Geometry: final body of the model. Coordinates: model frame, mm. Coordinates: 2 decimals unless noted, no trailing zeros. Order: outer loops, then holes, each group sorted by start corner. A loop starts at its lowest first (then second) coordinate and runs counter-clockwise, first axis right, second up. Notation, with made-up numbers: (-5.5, 28) -> (43.5, 28) arc R16 cw to (43.5, 51) -> close; hole circle Ø6 at (-20, -9.5). An arc over 180 degrees is marked (long way). Use one line per item in the form item = value.
```python
from build123d import *

# Parameters (mm, degrees)
EXTRUDE_1_DEPTH = 6


with BuildPart() as part:
    # 스케치1 → 보스-돌출1 (new, symmetric)
    with BuildSketch(Plane(origin=(0, 0, 0), x_dir=(0, 0, -1), z_dir=(1, 0, 0))):
        with BuildLine():
            Line((0, 6), (0, -6))
            Line((0, -6), (-60, -12))
            Line((-60, -12), (-70, -12))
            Line((-70, -12), (-70, -7))
            Line((-70, -7), (-82, -7))
            Line((-82, -7), (-89.403074012, -12))
            Line((-89.403074012, -12), (-149, -12))
            Line((-149, -12), (-149, -20))
            Line((-149, -20), (-199.739657381, -20))
            Line((-199.739657381, -20), (-235.816329231, 20))
            Line((-235.816329231, 20), (-160, 20))
            Line((-160, 20), (-160, 16.749981814))
            Line((-160, 16.749981814), (-156.437513639, 12))
            Line((-156.437513639, 12), (-156.019273901, 12))
            Line((-156.019273901, 12), (-153.375521927, 9.919487169))
            ThreePointArc((-153.375521927, 9.919487169), (-148.913971149, 8.215866364), (-146.000538153, 12))
            Line((-146.000538153, 12), (-60, 12))
            Line((-60, 12), (0, 6))
        make_face()
    extrude(amount=EXTRUDE_1_DEPTH, both=True)


solid = part.part
```
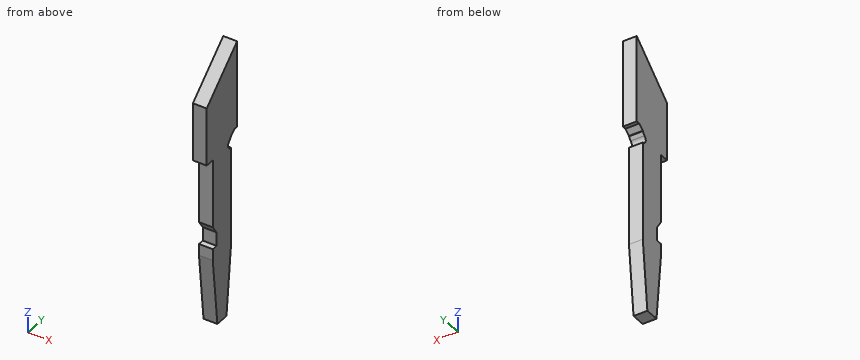
1) Section C-C, the plane y = 4. Output: boundary loops of the cut face in (x, z).
Results found:
outline = (-6, 0) -> (6, 0) -> (6, 221.39) -> (-6, 221.39) -> close
2) Section A-A, the plane x = -4. Output: boundary loops of the cut face in (y, z), and give its area (3 significant figures).
Results found:
outline = (-20, 149) -> (-12, 149) -> (-12, 89.4) -> (-7, 82) -> (-7, 70) -> (-12, 70) -> (-12, 60) -> (-6, 0) -> (6, 0) -> (12, 60) -> (12, 146) arc R4 cw to (9.92, 153.38) -> (12, 156.02) -> (12, 156.44) -> (16.75, 160) -> (20, 160) -> (20, 235.82) -> (-20, 199.74) -> close
area = 5,780 mm2
3) Section B-B, the plane z = 104.5. Output: boundary loops of the cut face in (x, y), and give its area (3 significant figures).
Results found:
outline = (-6, -12) -> (6, -12) -> (6, 12) -> (-6, 12) -> close
area = 288 mm2
4) Contact query for flat-ended pins moving along their axis: P1, Ø1.5, axis at x = -3, y = 10.5, coming from the +Z side; P2, Ø2.5, axis at x = -1.5, y = -15.5, coming from the -Z side; P3, Ø3.5, axis at x = -2.5, z = 118, coming from the -Y side. Output: stop coordinate, or through.
Results found:
P1 = 227.92
P2 = 149
P3 = -12
5) Material intervals for probe 1 along Y at (x, z) = (0.5, 117.5); probe 2 along Z at (x, y) = (2, 15); probe 3 along Z at (x, y) = (-3.25, 17.5), sorted ascending. Write a range as from..to.
Results found:
probe_1 = -12..12
probe_2 = 158.69..231.31
probe_3 = 160..233.56
